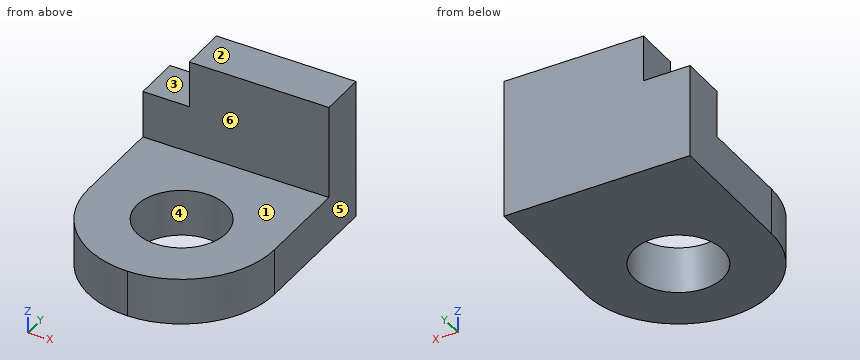
```python
from build123d import *

# Parameters (mm, degrees)
F0_W     = 50.8
F0_H     = 38.1
F1_DEPTH = 12.7
F2_W     = 12.7
F2_H     = 12.7
F3_DEPTH = 12.7
F4_W     = 50.8
F4_H     = 12.7
F5_DEPTH = 63.5
F6_R     = 12.14233
F7_DEPTH = 12.701


with BuildPart() as f1:
    # F0 (on Front) → F1 (new body)
    with BuildSketch(Plane.XZ):
        Rectangle(F0_W, F0_H)
    extrude(amount=F1_DEPTH)

    # F2 (on Front) → F3 (cut)
    with BuildSketch(Plane.XZ):
        with Locations((-19.05, 12.7)):
            Rectangle(F2_W, F2_H)
    extrude(amount=F3_DEPTH, mode=Mode.SUBTRACT)

    # F4 (on Front) → F5 (join)
    with BuildSketch(Plane.XZ):
        with Locations((0, -12.89534)):
            Rectangle(F4_W, F4_H)
    extrude(amount=F5_DEPTH)

    # F6 (on face) → F7 (cut, through all)
    with BuildSketch(Plane.XY.offset(-6.54534)):
        with BuildLine():
            Line((-25.4, -63.5), (0, -63.5))
            ThreePointArc((0, -63.5), (-17.960512, -56.060512), (-25.4, -38.1))
            Line((-25.4, -38.1), (-25.4, -63.5))
        make_face()
        with BuildLine():
            Line((25.4, -63.5), (25.4, -38.1))
            ThreePointArc((25.4, -38.1), (17.960512, -56.060512), (0, -63.5))
            Line((0, -63.5), (25.4, -63.5))
        make_face()
        with Locations((0, -38.1)):
            Circle(F6_R)
    extrude(amount=-F7_DEPTH, mode=Mode.SUBTRACT)


solid = f1.part
```
Part model, mm, in its own coordinate system. Face numbers are marked on the shaded views. A direction names the side the tool comes from. Round coordinates to 2 decimals unless told otherwise and drop trailing zeros. Write each loop counter-clockwise with the first axis right and the second up, starting at its lowest first coordinate (ties: lowest second). Pieces come first, ordered by that corner, then holes.
Item 1: Cut at A-A, the plane z = -10. Give the cut face in (x, y).
Results:
outline: (-25.4, -38.1) arc R25.4 ccw to (0, -63.5) arc R25.4 ccw to (25.4, -38.1) - (25.4, 0) - (-25.4, 0) - close; hole circle Ø24.28 at (0, -38.1)
Item 2: Cut at D-D, the plane y = -47.5. Give the cut face in (x, z), plus the area to 3 significant figures.
Results:
outline: (-23.6, -19.25) - (-7.69, -19.25) - (-7.69, -6.55) - (-23.6, -6.55) - close; (7.69, -19.25) - (23.6, -19.25) - (23.6, -6.55) - (7.69, -6.55) - close
area: 404 mm2
Item 3: Probe L1, parallel to Y at x = 0, z = -16.5; L2, parallel to Y at x = 0.5, z = 12; L3, parallel to Z at x = -10, y = -58.5. List the from-to ranges inside material, lowest first.
Results:
L1: y = -63.5 to -50.24, -25.96 to 0
L2: y = -12.7 to 0
L3: z = -19.25 to -6.55
Item 4: Which spindle directions (+Z, -Z, +X, -X, +Y, -Y) get a long thin tool onto all of the face, cutting with end or side? Do the marked faces 1, 2 and 3. Say none if no direction does.
Results:
face 1: +Z, +X, -X, -Y
face 2: +Z, +X, -X, +Y, -Y
face 3: +Z, -X, +Y, -Y
Item 5: Drop flat-ended pins along their axis: pin 1 Ø10 at (y, z) = (-36.5, 1.5) entering from -X; pin 2 Ø13 at (x, z) = (3.5, 5.5) entering from -Y; pin 3 Ø2 at (x, y) = (-15, -13.5) entering from +Z; pin 4 Ø5 at (x, z) = (-17.5, 4.5) entering from +Y. Give the stop position or say it passes through.
Results:
pin 1: passes through
pin 2: stops at y = -12.7
pin 3: stops at z = 6.35
pin 4: stops at y = 0
Item 6: Two-plate mould, pull along X, no slides. Class the marked faces 4, 5 and 6: +X half, -X half, draft (parallel to the pull), parting line (faces both ways), or undercut.
Results:
face 4: undercut
face 5: +X half
face 6: draft
Item 7: Cut at C-C, the plane y = -4. Give the cut face in (x, z).
Results:
outline: (-25.4, -19.25) - (25.4, -19.25) - (25.4, 19.05) - (-12.7, 19.05) - (-12.7, 6.35) - (-25.4, 6.35) - close
Item 8: Cut at B-B, the plane x = 9. Give the cut face in (y, z), plus the area to 3 significant figures.
Results:
outline: (-61.85, -19.25) - (-46.25, -19.25) - (-46.25, -6.55) - (-61.85, -6.55) - close; (-29.95, -19.25) - (0, -19.25) - (0, 19.05) - (-12.7, 19.05) - (-12.7, -6.55) - (-29.95, -6.55) - close
area: 904 mm2
